Source: CAD feature listing. Evaluate the final solid. Frame: model axes, mm. Face numbers are marked on the shaded views. A direction names the side the tool comes from. Round coordinates to 2 decimals unless told otherwise and drop trailing zeros. Loops run counter-clockwise (first coordinate to the right, second up) from the corner with the lowest first, then second, coordinate; pieces in that order, holes last.
Item 1: Ray query, L1, parallel to X at y = 7.75, z = 9.75; L2, parallel to X at y = 6, z = 8.75; L3, parallel to X at y = 0, z = 7. Return the intervals inside material, ascending.
Item 2: Section query A-A on x = 0. Return loops of the section in (y, z).
Item 3: Section query D-D on y = 9.75. Return loops of the section in (x, z), then the cut area to 3 significant figures.
Item 4: Section query B-B on y = -8.25. Return loops of the section in (x, z), then the cut area to 3 significant figures.
Item 5: First-contact query: P1, Ø5, axis at x = -2.5, y = 6, coming from the -Z side; P2, Ø0.7, axis at y = 13.5, z = 3.5, coming from the +X side; P3, Ø4, axis at y = 6.5, z = 4, coming from the +X side; P4, Ø1.5, axis at x = -5.5, z = 5.5, coming from the -Y side. Flat tips, straight axial feed; report the tip coordinate or a pass-through.
Item 6: Access query for the marked faces 4 and 5. Directions: +Z, -Z, +X, -X, +Y, -Y. A direction counts if a zero-diameter tool reaches every point of the face in a straight line with its end or side. Return the directions, or none.
Item 7: Section query C-C on y = -0.25. Return loops of the section in (x, z), then the cut area to 3 significant figures.
Item 8: Pull-direction query (Y, two-part tool) for the marked faces 1, 2 and 3; classes: released by +Y, released by -Y, zero draft, split by the parting line, or undercut.
```python
from build123d import *

# Parameters (mm, degrees)
SKETCH_1_R               = 4.1
EXTRUDE_1_DEPTH          = 10
CUT_EXTRUDE_1_DEPTH      = 10
PATTERN_CIRCULAR_1_COUNT = 3


with BuildPart() as part:
    # 草图1 → 凸台-拉伸1 (new body)
    with BuildSketch(Plane.XY):
        with BuildLine():
            Line((-3, 13.5), (-3, 12.905909499))
            ThreePointArc((-3, 12.905909499), (-11.4748366, 6.625), (-12.676845485, -3.854878538))
            Line((-12.676845485, -3.854878538), (-13.191342951, -4.151923789))
            Line((-13.191342951, -4.151923789), (-12.316342951, -5.667468245))
            ThreePointArc((-12.316342951, -5.667468245), (-10.608811196, -6.125), (-11.066342951, -7.832531755))
            Line((-11.066342951, -7.832531755), (-10.191342951, -9.348076211))
            Line((-10.191342951, -9.348076211), (-9.676845485, -9.051030961))
            ThreePointArc((-9.676845485, -9.051030961), (0, -13.25), (9.676845485, -9.051030961))
            Line((9.676845485, -9.051030961), (10.191342951, -9.348076211))
            Line((10.191342951, -9.348076211), (11.066342951, -7.832531755))
            ThreePointArc((11.066342951, -7.832531755), (10.608811196, -6.125), (12.316342951, -5.667468245))
            Line((12.316342951, -5.667468245), (13.191342951, -4.151923789))
            Line((13.191342951, -4.151923789), (12.676845485, -3.854878538))
            ThreePointArc((12.676845485, -3.854878538), (11.4748366, 6.625), (3, 12.905909499))
            Line((3, 12.905909499), (3, 13.5))
            Line((3, 13.5), (1.25, 13.5))
            ThreePointArc((1.25, 13.5), (0, 12.25), (-1.25, 13.5))
            Line((-1.25, 13.5), (-3, 13.5))
        make_face()
        Circle(SKETCH_1_R, mode=Mode.SUBTRACT)
    extrude(amount=EXTRUDE_1_DEPTH)

    # 草图2 → 切除-拉伸1 (cut)
    with BuildSketch(Plane.XY):
        with BuildLine():
            Line((-7.748999943, -6.78328828), (-3.470031597, -4.312824754))
            Line((-3.470031597, -4.312824754), (-1.025, -4.56980793))
            Line((-1.025, -4.56980793), (-1.025, -3.96980793))
            ThreePointArc((-1.025, -3.96980793), (0, -4.1), (1.025, -3.96980793))
            Line((1.025, -3.96980793), (1.025, -4.56980793))
            Line((1.025, -4.56980793), (3.470031597, -4.312824754))
            Line((3.470031597, -4.312824754), (7.748999943, -6.78328828))
            ThreePointArc((7.748999943, -6.78328828), (7.871108829, -6.961884233), (7.808154531, -7.168871796))
            ThreePointArc((7.808154531, -7.168871796), (0, -10.6), (-7.808154531, -7.168871796))
            ThreePointArc((-7.808154531, -7.168871796), (-7.871108829, -6.961884233), (-7.748999943, -6.78328828))
        make_face()
    cut_extrude_1 = extrude(amount=CUT_EXTRUDE_1_DEPTH, mode=Mode.SUBTRACT)

    # 阵列(圆周)1: 切除-拉伸1 ×3 about axis
    pattern_circular_1_axis = Axis((0, 0, 0), (0, 0, 1))
    for i in range(1, PATTERN_CIRCULAR_1_COUNT):
        add(cut_extrude_1.rotate(pattern_circular_1_axis, i * 360 / PATTERN_CIRCULAR_1_COUNT), mode=Mode.SUBTRACT)


solid = part.part
```
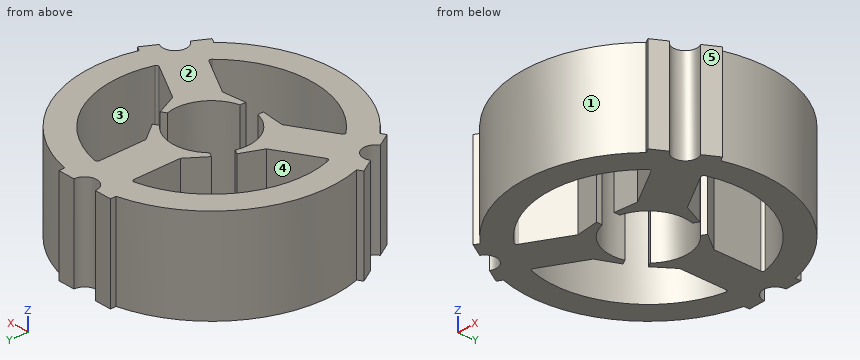
Data:
1. L1: x = -10.75 to -7.23, -2 to 2, 7.23 to 10.75
1. L2: x = -11.81 to -8.74, -2 to 2, 8.74 to 11.81
1. L3: x = -13.25 to -10.6, -5.09 to -4.1, 4.1 to 5.09, 10.6 to 13.25
2. outline: (-13.25, 0) - (-10.6, 0) - (-10.6, 10) - (-13.25, 10) - close; (4.1, 0) - (12.25, 0) - (12.25, 10) - (4.1, 10) - close
3. outline: (-8.97, 0) - (-4.16, 0) - (-4.16, 10) - (-8.97, 10) - close; (-2, 0) - (2, 0) - (2, 10) - (-2, 10) - close; (4.16, 0) - (8.97, 0) - (8.97, 10) - (4.16, 10) - close
3. area: 136 mm2
4. outline: (-10.83, 0) - (-6.66, 0) - (-6.66, 10) - (-10.83, 10) - close; (6.66, 0) - (10.83, 0) - (10.83, 10) - (6.66, 10) - close
4. area: 83.4 mm2
5. P1: stops at z = 0
5. P2: stops at x = 3
5. P3: stops at x = 12.46
5. P4: stops at y = -12.37
6. face 4: +Z, -Z
6. face 5: +Z, -Z, +X, -Y
7. outline: (-13.25, 0) - (-10.6, 0) - (-10.6, 10) - (-13.25, 10) - close; (-5.2, 0) - (-4.09, 0) - (-4.09, 10) - (-5.2, 10) - close; (4.09, 0) - (5.2, 0) - (5.2, 10) - (4.09, 10) - close; (10.6, 0) - (13.25, 0) - (13.25, 10) - (10.6, 10) - close
7. area: 75.2 mm2
8. face 1: released by -Y
8. face 2: zero draft
8. face 3: undercut
